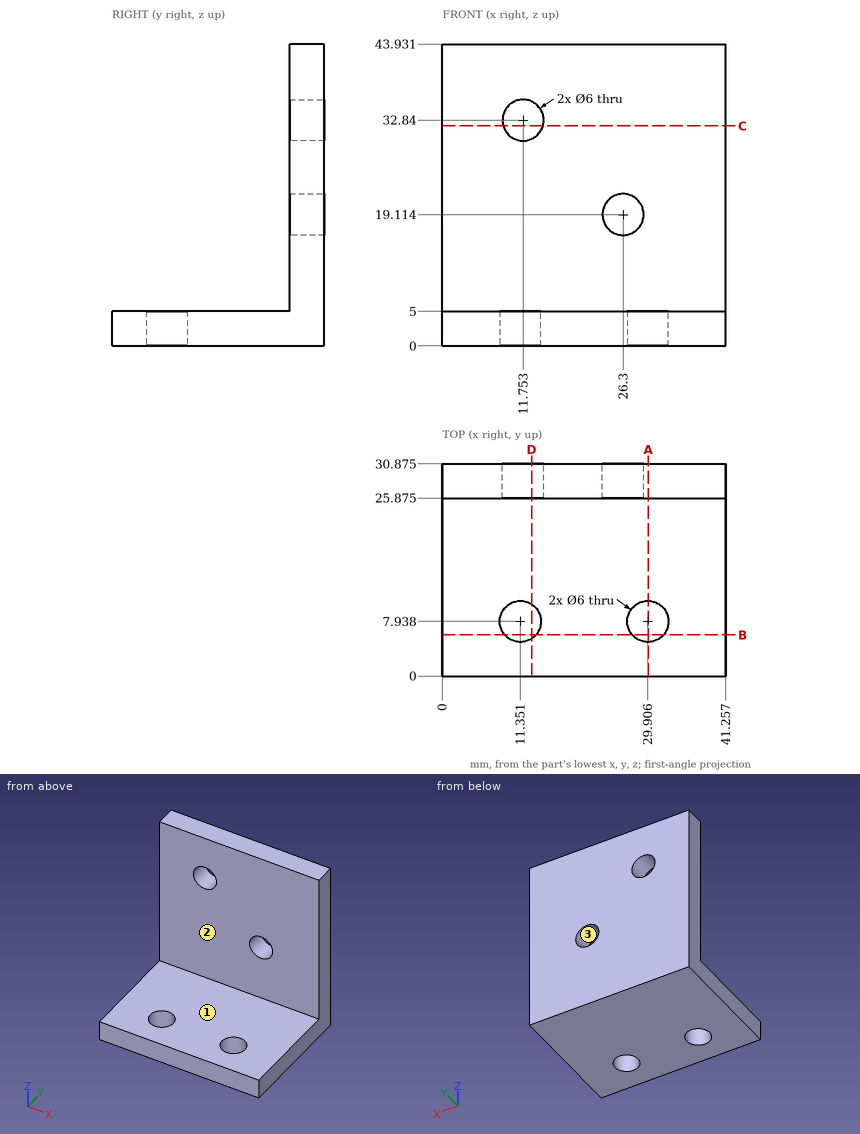
Here's the drawing with two shaded views (mm, measured from the low corner). I have some questions. Give positions to 0.01 mm unless a question says otherwise; leave off trailing zeros. Write each loop counter-clockwise with the first axis right and the second up, starting at its lowest first coordinate (ties: lowest second). Pieces come first, ordered by that corner, then holes. Notation, with made-up numbers: (88, 63) -> (103, 63) arc R12 cw to (103, 72) -> close; hole circle Ø11 at (48, 85.25). An arc over 180 degrees is marked (long way). Use one line per item in the form item = value. Start each with the question number.
1. Thinking about a two-plate mould opening in Z: for the marked faces 1, 2 and 3, which applies, +Z half, -Z half, draft (parallel to the pull), parting line (faces both ways), or undercut?
2. Will these pins go through, and if not, where does the flat tip stop? pin 1 Ø5 at (x, z) = (11.75, 32.84) entering from +Y; pin 2 Ø1.5 at (x, z) = (35.5, 25) entering from -Y (1 decimal); pin 3 Ø10 at (x, y) = (8.5, 17.5) entering from +Z.
3. Imagine slicing it at D-D on x = 13. List the corners of the cut face in (y, z) for me (1 decimal).
4. Imagine slicing it at C-C on z = 32. List the corners of the cut face in (x, y) for me (1 decimal).
5. If I drill on L1, parallel to Z at x = 37.5, y = 8; L2, parallel to Y at x = 21, z = 32.5 (1 decimal); L3, parallel to Z at x = 27, y = 28.5, over which ranges is the centre line in solid material (lowest first)?
6. Imagine slicing it at B-B on y = 6. List the corners of the cut face in (x, z) for me (1 decimal).
7. Imagine slicing it at A-A on x = 30. List the corners of the cut face in (y, z) for me (1 decimal).
Entries:
q1.face_1 = +Z half
q1.face_2 = draft
q1.face_3 = undercut
q2.pin_1 = through
q2.pin_2 = 25.9
q2.pin_3 = 5
q3.outline = (0, 0) -> (5.4, 0) -> (5.4, 5) -> (0, 5) -> close; (10.4, 0) -> (30.9, 0) -> (30.9, 30.1) -> (25.9, 30.1) -> (25.9, 5) -> (10.4, 5) -> close; (25.9, 35.6) -> (30.9, 35.6) -> (30.9, 43.9) -> (25.9, 43.9) -> close
q4.outline = (0, 25.9) -> (8.9, 25.9) -> (8.9, 30.9) -> (0, 30.9) -> close; (14.6, 25.9) -> (41.3, 25.9) -> (41.3, 30.9) -> (14.6, 30.9) -> close
q5.L1 = 0 to 5
q5.L2 = 25.9 to 30.9
q5.L3 = 0 to 16.2, 22.03 to 43.93
q6.outline = (0, 0) -> (9.1, 0) -> (9.1, 5) -> (0, 5) -> close; (13.6, 0) -> (27.6, 0) -> (27.6, 5) -> (13.6, 5) -> close; (32.2, 0) -> (41.3, 0) -> (41.3, 5) -> (32.2, 5) -> close
q7.outline = (0, 0) -> (4.9, 0) -> (4.9, 5) -> (0, 5) -> close; (10.9, 0) -> (30.9, 0) -> (30.9, 43.9) -> (25.9, 43.9) -> (25.9, 5) -> (10.9, 5) -> close
